from build123d import *

# Parameters (mm, degrees)
SKETCH1_W           = 50.8
SKETCH1_H           = 203.2
BOSS_EXTRUDE1_DEPTH = 3.175
SKETCH2_R           = 2.2
SKETCH2_R_2         = 2.159579804
SKETCH2_R_3         = 4
CUT_EXTRUDE1_DEPTH  = 10
SKETCH5_R           = 6
CUT_EXTRUDE2_DEPTH  = 10
CUT_EXTRUDE3_DEPTH  = 10


with BuildPart() as part:
    # Sketch1 → Boss-Extrude1 (new body)
    with BuildSketch(Plane(origin=(0, 0, 0), x_dir=(1, 0, 0), z_dir=(0, 1, 0))):
        with Locations((25.4, 101.6)):
            Rectangle(SKETCH1_W, SKETCH1_H)
    extrude(amount=BOSS_EXTRUDE1_DEPTH)

    # Sketch2 → Cut-Extrude1 (cut)
    with BuildSketch(Plane(origin=(0, 3.175, 0), x_dir=(1, 0, 0), z_dir=(0, 1, 0))):
        with Locations(Location((22.384513462, 187.103195302, 0), (0, 0, 270))):
            Circle(SKETCH2_R)
        with Locations(Location((38.36448905, 187.082300612, 0), (0, 0, 270))):
            Circle(SKETCH2_R_2)
        with Locations(Location((22.363364113, 170.92846049, 0), (0, 0, 270))):
            Circle(SKETCH2_R)
        with Locations(Location((38.343339701, 170.907565799, 0), (0, 0, 270))):
            Circle(SKETCH2_R_2)
        with Locations(Location((30.385513462, 179.103195302, 0), (0, 0, 270))):
            Circle(SKETCH2_R_3)
    extrude(amount=-CUT_EXTRUDE1_DEPTH, mode=Mode.SUBTRACT)

    # Sketch5 → Cut-Extrude2 (cut)
    with BuildSketch(Plane(origin=(0, 0, 0), x_dir=(-1, 0, 0), z_dir=(0, -1, 0))):
        with Locations(Location((-40.462848215, 9.36892711, 0), (0, 0, 90))):
            Circle(SKETCH5_R)
        with Locations(Location((-29.259232092, 118.036539738, 0), (0, 0, 90))):
            Circle(SKETCH5_R)
    extrude(amount=-CUT_EXTRUDE2_DEPTH, mode=Mode.SUBTRACT)

    # Sketch6 → Cut-Extrude3 (cut)
    with BuildSketch(Plane(origin=(0, 3.175, 0), x_dir=(1, 0, 0), z_dir=(0, 1, 0))):
        Polygon((0, 0), (19.29895822, 0), (-0.185019924, 105.431539045), align=None)
    extrude(amount=-CUT_EXTRUDE3_DEPTH, mode=Mode.SUBTRACT)


solid = part.part
Input: part model. Units: mm. Frame: model coordinates. Give positions to 0.01 mm unless a question says otherwise; leave off trailing zeros. Loops run counter-clockwise (first coordinate to the right, second up) from the corner with the lowest first, then second, coordinate; pieces in that order, holes last. Notation, with made-up numbers: (41.25, 75) -> (67.25, 75) arc R16 ccw to (67.25, 85) -> close; hole circle Ø8 at (-21, 5.5). An arc over 180 degrees is marked (long way). Answer as a JSON object with one key per item and string values. Group by question number.
Item 1: Line query: probe 1 along Z at (x, y) = (28.5, 2.45); probe 2 along Z at (x, y) = (27.5, 1.1); probe 3 along Z at (x, y) = (42.5, 1.2). Output: solid intervals per line, ascending.
Item 2: Cut plane A-A, the plane x = 43. Return the cut outline in (y, z) (3 decimals), and give its area (3 significant figures).
Item 3: Cut plane D-D, the plane z = -97. Return the cut outline in (x, y) (3 decimals).
Item 4: Cut plane B-B, the plane z = -119. Return the cut outline in (x, y) (3 decimals), and give its area (3 significant figures).
Item 5: Cut plane C-C, the plane y = 1.6. Return the cut outline in (x, z).
Item 6: Pin query (flat end, axial travel): P1, Ø7, axis at x = 30.39, z = -179.1, coming from the +Y side; P2, Ø1.5, axis at y = 2.5, z = -43, coming from the -X side. Return the tip coordinate at first contact, or that it passes through.
Item 7: Pull-direction query (Z, two-part tool) for faces 1 (the cylindrical face through (31.06, 1.57, -123.76)), 2 (the flat face through (25, 0, -103)), 3 (the flat face through (35, 2, 0)); classes: released by +Z, released by -Z, zero draft, split by the parting line, or undercut.
Checks:
{
 "1": {"probe 1": "z = -203.2 to -182.63, -175.58 to -123.99, -112.08 to 0", "probe 2": "z = -203.2 to -181.87, -176.33 to -123.77, -112.3 to 0", "probe 3": "z = -203.2 to -15.01, -3.73 to 0"},
 "2": {"outline": "(0, -203.2) -> (3.175, -203.2) -> (3.175, -14.806) -> (0, -14.806) -> close; (0, -3.932) -> (3.175, -3.932) -> (3.175, 0) -> (0, 0) -> close", "area": "611 mm²"},
 "3": {"outline": "(1.373, 0) -> (50.8, 0) -> (50.8, 3.175) -> (1.373, 3.175) -> close"},
 "4": {"outline": "(0, 0) -> (23.337, 0) -> (23.337, 3.175) -> (0, 3.175) -> close; (35.181, 0) -> (50.8, 0) -> (50.8, 3.175) -> (35.181, 3.175) -> close", "area": "124 mm²"},
 "5": {"outline": "(0, -203.2) -> (50.8, -203.2) -> (50.8, 0) -> (19.3, 0) -> (0, -104.43) -> close; hole circle Ø4.4 at (22.36, -170.93); hole circle Ø4.4 at (22.38, -187.1); hole circle Ø12 at (29.26, -118.04); hole circle Ø8 at (30.39, -179.1); hole circle Ø12 at (40.46, -9.37); hole circle Ø4.32 at (38.34, -170.91); hole circle Ø4.32 at (38.36, -187.08)"},
 "6": {"P1": "passes through", "P2": "stops at x = 11.21"},
 "7": {"face 1": "undercut", "face 2": "zero draft", "face 3": "released by +Z"}
}
